from build123d import *

# Parameters (mm, degrees)
CROQUIS1_R                        = 4
SALIENTE_EXTRUIR1_DEPTH           = 34
CORTAR_EXTRUIR1_REACH             = 36
CORTAR_EXTRUIR1_DIRECTION_2_REACH = 12
CORTAR_EXTRUIR2_REACH             = 72
CROQUIS4_R                        = 7.25


with BuildPart() as part:
    # Croquis1 → Saliente-Extruir1 (new body)
    with BuildSketch(Plane(origin=(17, 0, 0), x_dir=(0, 0, -1), z_dir=(1, 0, 0))):
        with BuildLine():
            Line((-10, 0), (-10, 60))
            Line((-10, 60), (34, 60))
            Line((34, 60), (9.323156657, -3.616455439))
            ThreePointArc((9.323156657, -3.616455439), (-1.839624069, -9.8293328), (-10, 0))
        make_face()
        Circle(CROQUIS1_R, mode=Mode.SUBTRACT)
    extrude(amount=-SALIENTE_EXTRUIR1_DEPTH)

    # Croquis3 → Cortar-Extruir1 (cut, up to next)
    with BuildSketch(Plane.XY, mode=Mode.PRIVATE) as cortar_extruir1_sk1:
        with BuildLine():
            Line((-15, -10), (15, -10))
            Line((15, -10), (15, 55))
            ThreePointArc((15, 55), (14.121320344, 57.121320344), (12, 58))
            Line((12, 58), (-12, 58))
            ThreePointArc((-12, 58), (-14.121320344, 57.121320344), (-15, 55))
            Line((-15, 55), (-15, -10))
        make_face()
    cortar_extruir1_tool1 = extrude(cortar_extruir1_sk1.sketch, amount=-CORTAR_EXTRUIR1_REACH, mode=Mode.PRIVATE) & part.part
    add(cortar_extruir1_tool1.solids().sort_by_distance((0, 23.936769, 0))[0], mode=Mode.SUBTRACT)

    # Croquis3 → Cortar-Extruir1 direction 2 (cut, up to next)
    with BuildSketch(Plane.XY, mode=Mode.PRIVATE) as cortar_extruir1_direction_2_sk1:
        with BuildLine():
            Line((-15, -10), (15, -10))
            Line((15, -10), (15, 55))
            ThreePointArc((15, 55), (14.121320344, 57.121320344), (12, 58))
            Line((12, 58), (-12, 58))
            ThreePointArc((-12, 58), (-14.121320344, 57.121320344), (-15, 55))
            Line((-15, 55), (-15, -10))
        make_face()
    cortar_extruir1_direction_2_tool1 = extrude(cortar_extruir1_direction_2_sk1.sketch, amount=CORTAR_EXTRUIR1_DIRECTION_2_REACH, mode=Mode.PRIVATE) & part.part
    add(cortar_extruir1_direction_2_tool1.solids().sort_by_distance((0, 23.936769, 0))[0], mode=Mode.SUBTRACT)

    # Croquis4 → Cortar-Extruir2 (cut, up to next)
    with BuildSketch(Plane(origin=(0, 60, 0), x_dir=(1, 0, 0), z_dir=(0, 1, 0)), mode=Mode.PRIVATE) as cortar_extruir2_sk1:
        with Locations((0, 12)):
            Circle(CROQUIS4_R)
    cortar_extruir2_tool1 = extrude(cortar_extruir2_sk1.sketch, amount=-CORTAR_EXTRUIR2_REACH, mode=Mode.PRIVATE) & part.part
    add(cortar_extruir2_tool1.solids().sort_by_distance((0, 60, -12))[0], mode=Mode.SUBTRACT)


solid = part.part
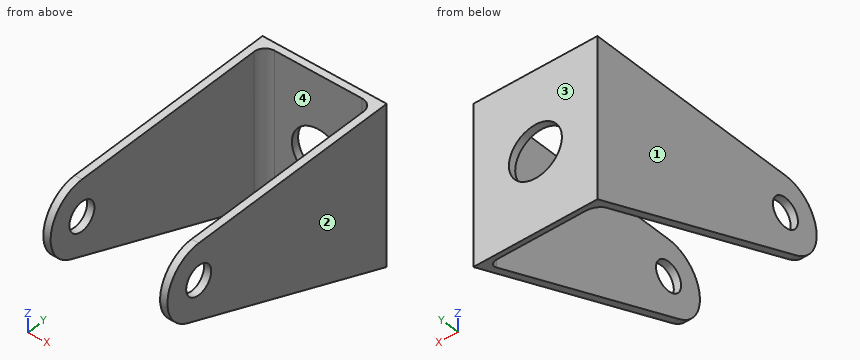
Geometry check sheet. Reference: the model listing, model coordinates, mm. Face numbers are marked on the shaded views. Round coordinates to 2 decimals unless told otherwise and drop trailing zeros. Loops run counter-clockwise (first coordinate to the right, second up) from the corner with the lowest first, then second, coordinate; pieces in that order, holes last.
Item 1: Cross-section at C-C on y = 44.5. Record the boundary of the cut face in (x, z).
Item 2: Cross-section at A-A on x = -5. Record the boundary of the cut face in (y, z).
Item 3: Cross-section at D-D on z = -12. Record the boundary of the cut face in (x, y).
Item 4: Gauge pin test, flat ends, axial feed: pin 1 (1.5 mm diameter, centred on x = -2, z = -18, fed in from +Y); pin 2 (7 mm diameter, centred on x = 2, z = -3.5, fed in from -Y). Record the tip position at first contact, or that the pin passes through.
Item 5: Mould release check, pull along X, two halves, no side actions. Record for the marked faces 1, 2, 3 and 4: pulls with the +X half, pulls with the -X half, needs draft (parallel to the pull), parting line crosses it, or undercut.
Item 6: Cross-section at B-B on z = 0. Record the boundary of the cut face in (x, y), then the cut area to 3 significant figures.
Item 7: Thickness scan on line 1 (Y direction, x = 16, z = 0); line 2 (X direction, y = 12, z = 5.5); line 3 (X direction, y = 58.75, z = -12). Record the ranges inside material, lowest first.
Answer sheet:
1. outline: (-17, -27.99) - (-15, -27.99) - (-15, 10) - (-17, 10) - close; (15, -27.99) - (17, -27.99) - (17, 10) - (15, 10) - close
2. outline: (58, -33.22) - (60, -34) - (60, -17.25) - (58, -17.25) - close; (58, -6.75) - (60, -6.75) - (60, 10) - (58, 10) - close
3. outline: (-17, 3.28) - (-15, 3.28) - (-15, 55) arc R3 cw to (-12, 58) - (-7.25, 58) - (-7.25, 60) - (-17, 60) - close; (7.25, 58) - (12, 58) arc R3 cw to (15, 55) - (15, 3.28) - (17, 3.28) - (17, 60) - (7.25, 60) - close
4. pin 1: passes through
4. pin 2: stops at y = 58
5. face 1: pulls with the -X half
5. face 2: pulls with the +X half
5. face 3: needs draft
5. face 4: undercut
6. outline: (-17, -10) - (-15, -10) - (-15, -4) - (-17, -4) - close; (-17, 4) - (-15, 4) - (-15, 55) arc R3 cw to (-12, 58) - (12, 58) arc R3 cw to (15, 55) - (15, 4) - (17, 4) - (17, 60) - (-17, 60) - close; (15, -10) - (17, -10) - (17, -4) - (15, -4) - close
6. area: 312 mm2
7. line 1: y = -10 to -4, 4 to 60
7. line 2: x = -17 to -15, 15 to 17
7. line 3: x = -17 to -7.25, 7.25 to 17
